```python
from build123d import *

# Parameters (mm, degrees)
SKETCH_1_W          = 40
SKETCH_1_H          = 40
EXTRUDE_1_DEPTH     = 10
FILLET_1_R          = 2
CUT_EXTRUDE_1_DEPTH = 8
FILLET_2_R          = 2
SKETCH_3_R          = 1.5
SKETCH_3_R_2        = 1.4999999999999978
SKETCH_3_R_3        = 1.500000000000004
SKETCH_3_R_4        = 1.5000000000000042
CUT_EXTRUDE_2_DEPTH = 58.445626465380286
CUT_EXTRUDE_3_DEPTH = 58.445626465380286
FILLET_3_R          = 2


with BuildPart() as part:
    # 草图1 → 凸台-拉伸1 (new body)
    with BuildSketch(Plane(origin=(0, 0, 0), x_dir=(1, 0, 0), z_dir=(0, 1, 0))):
        with Locations((20, 20)):
            Rectangle(SKETCH_1_W, SKETCH_1_H)
    extrude(amount=EXTRUDE_1_DEPTH)

    # 圆角1
    fillet_1_edges = [part.edges().sort_by_distance(p)[0] for p in [
        (0, 5, -40),
        (40, 5, -40),
        (40, 5, 0),
        (0, 5, 0),
    ]]
    fillet(fillet_1_edges, radius=FILLET_1_R)

    # 草图2 → 切除-拉伸1 (cut)
    with BuildSketch(Plane(origin=(0, 10, 0), x_dir=(1, 0, 0), z_dir=(0, 1, 0))):
        Polygon((6, 5.999999999999999), (34, 6), (34, 34), (5.999999999999999, 34), align=None)
    extrude(amount=-CUT_EXTRUDE_1_DEPTH, mode=Mode.SUBTRACT)

    # 圆角2
    fillet_2_edges = [part.edges().sort_by_distance(p)[0] for p in [
        (6, 6, -5.999999999999999),
        (5.999999999999999, 6, -34),
        (34, 6, -34),
        (34, 6, -6),
    ]]
    fillet(fillet_2_edges, radius=FILLET_2_R)

    # 草图3 → 切除-拉伸2 (cut, through all)
    with BuildSketch(Plane(origin=(0, 10, 0), x_dir=(1, 0, 0), z_dir=(0, 1, 0))):
        with Locations(Location((4.0000000000000036, 36.00000000000001, 0), (0, 0, 270))):
            Circle(SKETCH_3_R)
        with Locations(Location((4.0000000000000036, 4, 0), (0, 0, 90))):
            Circle(SKETCH_3_R_2)
        with Locations(Location((36.00000000000001, 4.000000000000004, 0), (0, 0, 270))):
            Circle(SKETCH_3_R_3)
        with Locations(Location((36.00000000000001, 36.00000000000002, 0), (0, 0, 90))):
            Circle(SKETCH_3_R_4)
    extrude(amount=-CUT_EXTRUDE_2_DEPTH, mode=Mode.SUBTRACT)

    # 草图4 → 切除-拉伸3 (cut, through all)
    with BuildSketch(Plane.XZ):
        with BuildLine():
            ThreePointArc((21.923076923076923, -24.615384615384617), (18.815219099044967, -24.857601693915647), (16.167883211678838, -23.211678832116792))
            Line((16.167883211678838, -23.211678832116792), (2.9999999999999947, -7.5))
            Line((2.999999999999995, -7.5), (2.999999999999995, -32.5))
            Line((2.9999999999999964, -32.5), (21.923076923076927, -24.615384615384624))
        make_face()
        with BuildLine():
            Line((7.500000000000055, -2.9999999999999467), (15.38461538461537, -21.923076923076906))
            ThreePointArc((15.384615384615378, -21.923076923076902), (15.14239830608436, -18.815219099044945), (16.788321167883222, -16.167883211678824))
            Line((16.788321167883222, -16.167883211678824), (32.50000000000006, -3.0000000000000355))
            Line((32.50000000000006, -3.000000000000034), (7.500000000000057, -2.9999999999999467))
        make_face()
        with BuildLine():
            Line((37.0000000000001, -7.500000000000116), (18.076923076923116, -15.384615384615365))
            ThreePointArc((18.07692307692312, -15.384615384615369), (21.184780900955076, -15.14239830608436), (23.832116788321194, -16.788321167883236))
            Line((23.832116788321194, -16.788321167883232), (36.99999999999993, -32.50000000000012))
            Line((36.99999999999993, -32.50000000000012), (37.0000000000001, -7.500000000000117))
        make_face()
        with BuildLine():
            ThreePointArc((25.000000000000004, -20), (24.53091569997632, -22.114427326655647), (23.211678832116753, -23.8321167883212))
            Line((23.211678832116757, -23.832116788321205), (7.499999999999826, -36.99999999999988))
            Line((7.499999999999827, -36.99999999999988), (32.49999999999984, -37.00000000000014))
            Line((32.49999999999984, -37.00000000000014), (24.615384615384645, -18.07692307692313))
            ThreePointArc((24.61538461538464, -18.07692307692313), (24.90290337845461, -19.01941932430911), (25.000000000000004, -20))
        make_face()
    extrude(amount=-CUT_EXTRUDE_3_DEPTH, mode=Mode.SUBTRACT)

    # 圆角3
    fillet_3_edges = [part.edges().sort_by_distance(p)[0] for p in [
        (18.076923076923116, 1, -15.384615384615367),
        (15.384615384615376, 1, -21.923076923076906),
        (24.61538461538464, 1, -18.07692307692313),
    ]]
    fillet(fillet_3_edges, radius=FILLET_3_R)
    fillet_3_2_edges = [part.edges().sort_by_distance(p)[0] for p in [
        (21.923076923076927, 1, -24.61538461538462),
    ]]
    fillet(fillet_3_2_edges, radius=FILLET_3_R - 0.0001)  # a hair under: the kernel refuses the full size


solid = part.part
```
Check sheet for the modelled part. Datum: model origin and axes. Units: mm. A direction names the side the tool comes from. Coordinates: 2 decimals unless noted, no trailing zeros. Loops run counter-clockwise (first coordinate to the right, second up) from the corner with the lowest first, then second, coordinate; pieces in that order, holes last.
1) Material ranges on probe 1 along Z at (x, y) = (15, 5.5); probe 2 along X at (y, z) = (4.25, -4); probe 3 along X at (y, z) = (6, -17.5), recorded low to high.
2) Sectioned sample at B-B (y = 0.75). Count the separate pieces of the cut face and the enclosed holes in it, and give its area (3 significant figures).
3) Release check for a two-part mould opening along X. For faces 4 (the face through (14.43, 1.01, -17.28)), 5 (the face through (39.4, 5.07, -0.57)), 6 (the face through (20, 5, 0)) record: released by +X, released by -X, zero draft, split by the parting line, or undercut.
4) Gauge pin test, flat end, axial feed: pin 1 (2.5 mm diameter, centred on x = 36, z = -4, fed in from -Y). Record the tip position at first contact, or that the pin passes through.
5) Sectioned sample at C-C (z = -4). Record the boundary of the cut face in (x, y).
6) Sectioned sample at A-A (z = -33.5). Record the boundary of the cut face in (x, y).
7) Sectioned sample at D-D (x = 18.5). Record the boundary of the cut face in (y, z), and give its area (3 significant figures).
8) Access from +Z, -Z, +X, -X, +Y, -Y to the whole of each face (thin tool, end or side, straight path). Record for faces 1 (the face through (20, 0, -20)), 2 (the face through (11.974, 1.597, -33.25)), 3 (the face through (30, 6, -6)).
Check sheet entries:
1. probe 1: z = -40 to -37, -3 to 0
1. probe 2: x = 0 to 2.5, 5.5 to 7.92, 31.31 to 34.5, 37.5 to 40
1. probe 3: x = 0 to 3, 37 to 40
2. separate pieces: 1
2. enclosed holes: 8
2. area: 798 mm2
3. face 4: undercut
3. face 5: released by +X
3. face 6: zero draft
4. pin 1: passes through
5. outline: (0, 0) - (2.5, 0) - (2.5, 10) - (0, 10) - close; (5.5, 0) - (7.92, 0) - (7.92, 10) - (5.5, 10) - close; (31.31, 0) - (34.5, 0) - (34.5, 10) - (31.31, 10) - close; (37.5, 0) - (40, 0) - (40, 10) - (37.5, 10) - close
6. outline: (0, 0) - (11.68, 0) - (11.68, 2) - (6.68, 2) - (6.68, 10) - (0, 10) - close; (31.04, 0) - (40, 0) - (40, 10) - (33.32, 10) - (33.32, 2) - (31.04, 2) - close
7. outline: (0, -40) - (10, -40) - (10, -37) - (0, -37) - close; (0, -27.78) - (2, -27.78) - (2, -14.73) - (0, -14.73) - close; (0, -3) - (10, -3) - (10, 0) - (0, 0) - close
7. area: 86.1 mm2
8. face 1: +Z, -Z, +X, -X, -Y
8. face 2: +Y, -Y
8. face 3: +Y
